Read the model definition and answer for the solid it produces. Units are mm, in the model's axes. Coordinates: 2 decimals unless noted, no trailing zeros. Write each loop counter-clockwise with the first axis right and the second up, starting at its lowest first coordinate (ties: lowest second). Pieces come first, ordered by that corner, then holes.
(1) Section C-C on z = 4 is taken. Write down the section's boundary in (x, y).
(2) Section A-A on y = 152.4 is taken. Write down the section's boundary in (x, z), then the cut area to 3 significant figures.
(3) Find the intervals of material crossed by probe 1 along Y at (x, z) = (152.4, 4.75); probe 2 along Y at (x, z) = (75.5, 4.5); probe 3 along X at (y, z) = (239, 6.25), in increasing order.
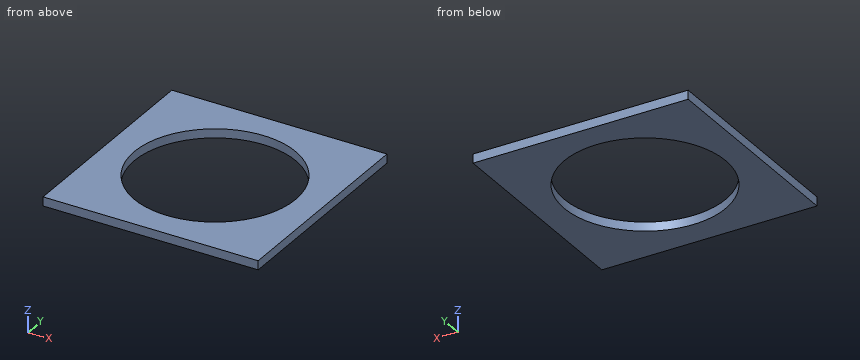
Autodesk Inventor part; units mm, degrees
ref_plane "YZ Plane" through (0, 0, 0) normal (1, 0, 0) x (0, 1, 0)
ref_plane "XZ Plane" through (0, 0, 0) normal (0, 1, 0) x (-1, 0, 0)
ref_plane "XY Plane" through (0, 0, 0) normal (0, 0, 1) x (1, 0, 0)
sketch "Sketch1" plane through (0, 0, 0) normal (0, 0, 1) x (1, 0, 0)
  line L0 (0, 0) -> (304.8, 0)
  line L1 (304.8, 0) -> (304.8, 304.8)
  line L2 (304.8, 304.8) -> (0, 304.8)
  line L3 (0, 304.8) -> (0, 0)
  circle A0 centre (152.4, 152.4) radius 114.3
  point P0 (304.8, 152.4)
  point P1 (152.4, 304.8)
  dimension "d0" = 304.8
  dimension "d1" = 228.6
extrude "Extrusion1" add sketch "Sketch1" along normal blind 12.7
properties material "MDF Medium Density Fiberboard"
Response:
1. outline: (0, 0) - (304.8, 0) - (304.8, 304.8) - (0, 304.8) - close; hole circle Ø228.6 at (152.4, 152.4)
2. outline: (0, 0) - (38.1, 0) - (38.1, 12.7) - (0, 12.7) - close; (266.7, 0) - (304.8, 0) - (304.8, 12.7) - (266.7, 12.7) - close
2. area: 968 mm2
3. probe 1: y = 0 to 38.1, 266.7 to 304.8
3. probe 2: y = 0 to 67.84, 236.96 to 304.8
3. probe 3: x = 0 to 77.8, 227 to 304.8
